Build history of the part. All positions in model axes, mm. Give positions to 0.01 mm unless a question says otherwise; leave off trailing zeros. Loops run counter-clockwise (first coordinate to the right, second up) from the corner with the lowest first, then second, coordinate; pieces in that order, holes last. Notation, with made-up numbers: M -17,86.5 L 3,86.5 A4 cw 3,92.5 Z; hole C 85,-25.75 d4. An arc over 180 degrees is marked long. Answer as a JSON object with one key per item and string values. Group by question number.
1. Mould opens along Z. For faces 1 (the face through (38, 0, -464)), 2 (the face through (48.39, 1.61, -827.35)) say: released by +Z, released by -Z, zero draft, split by the parting line, or undercut.
2. Drop flat-ended pins along their axis: pin 1 Ø6 at (x, z) = (21, -494.5) entering from -Y; pin 2 Ø18 at (x, z) = (50.8, -838.2) entering from +Y. Give the stop position or say it passes through.
3. Slice it at B-B (y = 1.6). List the corners of the cut face in (x, z) (1 decimal), then the cut area to 3 significant figures.
4. Slice it at A-A (z = -76.2). List the corners of the cut face in (x, y) (1 decimal), then the cut area to 3 significant figures.
5. Slice it at C-C (x = 50.8). List the corners of the cut face in (y, z) (1 decimal), then the cut area to 3 significant figures.
6. Drill centre lines: line 1 along Z through (x, y) = (50.8, 2.2); line 2 along X through (y, z) = (1.9, -76.2); line 3 along Z through (x, y) = (42, 0.15). Where is each one in solid material? Low to high. Write a range as [from, to].
from build123d import *

# Parameters (mm, degrees)
SKETCH1_W           = 76.2
SKETCH1_H           = 914.4
BOSS_EXTRUDE1_DEPTH = 3.175
CUT_EXTRUDE1_REACH  = 5.175
SKETCH2_R           = 11.1125


with BuildPart() as part:
    # Sketch1 → Boss-Extrude1 (new body)
    with BuildSketch(Plane(origin=(0, 0, 0), x_dir=(1, 0, 0), z_dir=(0, 1, 0))):
        with Locations((38.1, 457.2)):
            Rectangle(SKETCH1_W, SKETCH1_H)
    extrude(amount=BOSS_EXTRUDE1_DEPTH)

    # Sketch2 → Cut-Extrude1 (cut, up to next)
    with BuildSketch(Plane(origin=(0, 3.175, 0), x_dir=(1, 0, 0), z_dir=(0, 1, 0)), mode=Mode.PRIVATE) as cut_extrude1_sk1:
        with Locations((50.8, 838.2)):
            Circle(SKETCH2_R)
    cut_extrude1_tool1 = extrude(cut_extrude1_sk1.sketch, amount=-CUT_EXTRUDE1_REACH, mode=Mode.PRIVATE) & part.part
    add(cut_extrude1_tool1.solids().sort_by_distance((50.8, 3.175, -838.2))[0], mode=Mode.SUBTRACT)
    # Sketch2 → Cut-Extrude1 (cut, up to next)
    with BuildSketch(Plane(origin=(0, 3.175, 0), x_dir=(1, 0, 0), z_dir=(0, 1, 0)), mode=Mode.PRIVATE) as cut_extrude1_sk2:
        with Locations((50.8, 457.2)):
            Circle(SKETCH2_R)
    cut_extrude1_tool2 = extrude(cut_extrude1_sk2.sketch, amount=-CUT_EXTRUDE1_REACH, mode=Mode.PRIVATE) & part.part
    add(cut_extrude1_tool2.solids().sort_by_distance((50.8, 3.175, -457.2))[0], mode=Mode.SUBTRACT)
    # Sketch2 → Cut-Extrude1 (cut, up to next)
    with BuildSketch(Plane(origin=(0, 3.175, 0), x_dir=(1, 0, 0), z_dir=(0, 1, 0)), mode=Mode.PRIVATE) as cut_extrude1_sk3:
        with Locations((50.8, 76.2)):
            Circle(SKETCH2_R)
    cut_extrude1_tool3 = extrude(cut_extrude1_sk3.sketch, amount=-CUT_EXTRUDE1_REACH, mode=Mode.PRIVATE) & part.part
    add(cut_extrude1_tool3.solids().sort_by_distance((50.8, 3.175, -76.2))[0], mode=Mode.SUBTRACT)


solid = part.part
Established:
{
 "1": {"face 1": "zero draft", "face 2": "undercut"},
 "2": {"pin 1": "stops at y = 0", "pin 2": "passes through"},
 "3": {"outline": "M 0,-914.4 L 76.2,-914.4 L 76.2,0 L 0,0 Z; hole C 50.8,-838.2 d22.2; hole C 50.8,-457.2 d22.2; hole C 50.8,-76.2 d22.2", "area": "68,500 mm^2"},
 "4": {"outline": "M 0,0 L 39.7,0 L 39.7,3.2 L 0,3.2 Z; M 61.9,0 L 76.2,0 L 76.2,3.2 L 61.9,3.2 Z", "area": "171 mm^2"},
 "5": {"outline": "M 0,-914.4 L 3.2,-914.4 L 3.2,-849.3 L 0,-849.3 Z; M 0,-827.1 L 3.2,-827.1 L 3.2,-468.3 L 0,-468.3 Z; M 0,-446.1 L 3.2,-446.1 L 3.2,-87.3 L 0,-87.3 Z; M 0,-65.1 L 3.2,-65.1 L 3.2,0 L 0,0 Z", "area": "2,690 mm^2"},
 "6": {"line 1": "z = [-914.4, -849.31], [-827.09, -468.31], [-446.09, -87.31], [-65.09, 0]", "line 2": "x = [0, 39.69], [61.91, 76.2]", "line 3": "z = [-914.4, -844.99], [-831.41, -463.99], [-450.41, -82.99], [-69.41, 0]"}
}
